from build123d import *

# Parameters (mm, degrees)
F0_W         = 177.8
F0_H         = 304.8
F1_DEPTH     = 762
F3_DEPTH     = 12.7
F5_T1_DEPTH  = 279.4
F5_T3_DEPTH  = 152.4
F5_T5_DEPTH  = 781.05
F5_T7_DEPTH  = 206.9983323097
F5_S11_W     = 12.954
F5_S11_H     = 12.954
F5_T12_DEPTH = 12.954
F5_S17_W     = 12.954
F5_S17_H     = 12.954
F5_T18_DEPTH = 12.954
F5_S23_W     = 12.954
F5_S23_H     = 12.954
F5_T24_DEPTH = 12.954
F5_S29_W     = 12.954
F5_S29_H     = 12.954
F5_T30_DEPTH = 12.954
F5_T34_ANGLE = 180
F5_T36_ANGLE = 180
F5_T38_ANGLE = 160.6620429302
F5_T40_ANGLE = 121.9975948725
F5_T42_ANGLE = 121.9975948725


# Not quite as in the source:
# - a fillet or chamfer that OpenCascade refuses, or shapes differently, is made with other operations: its cross-section is extruded or revolved along the edge and cut away or added
# - a feature of the source that left no trace in its solid (it failed there, or was rolled back) is left out


with BuildPart() as f1:
    # F0 (on Top) → F1 (new body)
    with BuildSketch(Plane.XY):
        Rectangle(F0_W, F0_H)
    extrude(amount=F1_DEPTH)

    # F2 (on face) → F3 (join)
    with BuildSketch(Plane.XZ.offset(152.4)):
        with BuildLine():
            ThreePointArc((0, 190.5), (-61.5022268, 124.3675088832), (-63.5, 34.0788651625))
            ThreePointArc((-63.5, 34.0788651625), (-36.0333838653, 9.0580961901), (3.12e-07, 0))
            ThreePointArc((3.12e-07, 0), (36.0333841402, 9.0580963377), (63.5, 34.0788651625))
            ThreePointArc((63.5, 34.0788651625), (61.5022268, 124.3675088832), (0, 190.5))
        make_face()
        with BuildLine():
            ThreePointArc((63.5, 685.8), (0, 749.3), (-63.5, 685.8))
            Line((-63.5, 685.8), (-63.5, 478.8016676903))
            ThreePointArc((-63.5, 478.8016676903), (0, 415.3016676903), (63.5, 478.8016676903))
            Line((63.5, 478.8016676903), (63.5, 685.8))
        make_face()
    extrude(amount=F3_DEPTH)

    # F5: fillet of radius 12.7 on 15 edges, made by hand

    # F5_s2 → F5_t1 (cut)
    with BuildSketch(Plane.XZ.offset(-139.7)):
        with BuildLine():
            ThreePointArc((88.9, 749.3), (85.1802561211, 758.2802561211), (76.2, 762))
            Line((76.2, 762), (88.9, 762))
            Line((88.9, 762), (88.9, 749.3))
        make_face()
        with BuildLine():
            ThreePointArc((-76.2, 762), (-85.1802561211, 758.2802561211), (-88.9, 749.3))
            Line((-88.9, 749.3), (-88.9, 762))
            Line((-88.9, 762), (-76.2, 762))
        make_face()
    extrude(amount=F5_T1_DEPTH, mode=Mode.SUBTRACT)

    # F5_s4 → F5_t3 (cut)
    with BuildSketch(Plane.YZ.offset(-76.2)):
        with BuildLine():
            ThreePointArc((152.4, 749.3), (148.6802561211, 758.2802561211), (139.7, 762))
            Line((139.7, 762), (152.4, 762))
            Line((152.4, 762), (152.4, 749.3))
        make_face()
        with BuildLine():
            ThreePointArc((-152.4, 749.3), (-148.6802561211, 758.2802561211), (-139.7, 762))
            Line((-139.7, 762), (-152.4, 762))
            Line((-152.4, 762), (-152.4, 749.3))
        make_face()
    extrude(amount=F5_T3_DEPTH, mode=Mode.SUBTRACT)

    # F5_s6 → F5_t5 (cut)
    with BuildSketch(Plane.XY.offset(-31.75)):
        with BuildLine():
            ThreePointArc((-76.2, -152.4), (-85.1802561211, -148.6802561211), (-88.9, -139.7))
            Line((-88.9, -139.7), (-88.9, -152.4))
            Line((-88.9, -152.4), (-76.2, -152.4))
        make_face()
        with BuildLine():
            ThreePointArc((-76.2, 152.4), (-85.1802561211, 148.6802561211), (-88.9, 139.7))
            Line((-88.9, 139.7), (-88.9, 152.4))
            Line((-88.9, 152.4), (-76.2, 152.4))
        make_face()
        with BuildLine():
            ThreePointArc((88.9, -139.7), (85.1802561211, -148.6802561211), (76.2, -152.4))
            Line((76.2, -152.4), (88.9, -152.4))
            Line((88.9, -152.4), (88.9, -139.7))
        make_face()
        with BuildLine():
            ThreePointArc((88.9, 139.7), (85.1802561211, 148.6802561211), (76.2, 152.4))
            Line((76.2, 152.4), (88.9, 152.4))
            Line((88.9, 152.4), (88.9, 139.7))
        make_face()
    extrude(amount=F5_T5_DEPTH, mode=Mode.SUBTRACT)

    # F5_s8 → F5_t7 (cut)
    with BuildSketch(Plane.XY.offset(478.8016676903)):
        with BuildLine():
            ThreePointArc((63.5, -152.4), (59.7802561211, -161.3802561211), (50.8, -165.1))
            Line((50.8, -165.1), (63.5, -165.1))
            Line((63.5, -165.1), (63.5, -152.4))
        make_face()
        with BuildLine():
            ThreePointArc((-63.5, -152.4), (-59.7802561211, -161.3802561211), (-50.8, -165.1))
            Line((-50.8, -165.1), (-63.5, -165.1))
            Line((-63.5, -165.1), (-63.5, -152.4))
        make_face()
    extrude(amount=F5_T7_DEPTH, mode=Mode.SUBTRACT)


with BuildPart() as f5_tool10:
    # F5_s11 → F5_t12 (new body)
    with BuildSketch(Plane.YZ.offset(76.2)):
        with Locations((-146.177, 755.777)):
            Rectangle(F5_S11_W, F5_S11_H)
    extrude(amount=F5_T12_DEPTH)

    # F5_s13 → F5_t14 (revolve, cut)
    with BuildSketch(Plane(origin=(76.2, -139.7, 749.3), x_dir=(0, 0.7071067812, -0.7071067812), z_dir=(0, -0.7071067812, -0.7071067812))):
        with BuildLine():
            ThreePointArc((0, -12.7), (12.7, 0), (0, 12.7))
            Line((0, 12.7), (0, -12.7))
        make_face()
    revolve(axis=Axis((76.2, -139.7, 749.3), (1, 0, 0)), mode=Mode.SUBTRACT)


with BuildPart() as f1_1:
    add(f1.part)

    # F5_t9: cut F5_tool10
    add(f5_tool10.part, mode=Mode.SUBTRACT)


with BuildPart() as f5_tool16:
    # F5_s17 → F5_t18 (new body)
    with BuildSketch(Plane.YZ.offset(76.2)):
        with Locations((146.177, 755.777)):
            Rectangle(F5_S17_W, F5_S17_H)
    extrude(amount=F5_T18_DEPTH)

    # F5_s19 → F5_t20 (revolve, cut)
    with BuildSketch(Plane(origin=(76.2, 139.7, 749.3), x_dir=(0, -0.7071067812, -0.7071067812), z_dir=(0, -0.7071067812, 0.7071067812))):
        with BuildLine():
            ThreePointArc((0, -12.7), (12.7, 0), (0, 12.7))
            Line((0, 12.7), (0, -12.7))
        make_face()
    revolve(axis=Axis((76.2, 139.7, 749.3), (1, 0, 0)), mode=Mode.SUBTRACT)


with BuildPart() as f1_2:
    add(f1_1.part)

    # F5_t15: cut F5_tool16
    add(f5_tool16.part, mode=Mode.SUBTRACT)


with BuildPart() as f5_tool22:
    # F5_s23 → F5_t24 (new body)
    with BuildSketch(Plane.XZ.offset(-139.7)):
        with Locations((-82.677, 755.777)):
            Rectangle(F5_S23_W, F5_S23_H)
    extrude(amount=-F5_T24_DEPTH)

    # F5_s25 → F5_t26 (revolve, cut)
    with BuildSketch(Plane(origin=(-76.2, 139.7, 749.3), x_dir=(0.7071067812, 0, -0.7071067812), z_dir=(0.7071067812, 0, 0.7071067812))):
        with BuildLine():
            ThreePointArc((0, -12.7), (12.7, 0), (0, 12.7))
            Line((0, 12.7), (0, -12.7))
        make_face()
    revolve(axis=Axis((-76.2, 139.7, 749.3), (0, 1, 0)), mode=Mode.SUBTRACT)


with BuildPart() as f1_3:
    add(f1_2.part)

    # F5_t21: cut F5_tool22
    add(f5_tool22.part, mode=Mode.SUBTRACT)


with BuildPart() as f5_tool28:
    # F5_s29 → F5_t30 (new body)
    with BuildSketch(Plane.XZ.offset(139.7)):
        with Locations((-82.677, 755.777)):
            Rectangle(F5_S29_W, F5_S29_H)
    extrude(amount=F5_T30_DEPTH)

    # F5_s31 → F5_t32 (revolve, cut)
    with BuildSketch(Plane(origin=(-76.2, -139.7, 749.3), x_dir=(0.7071067812, 0, -0.7071067812), z_dir=(-0.7071067812, 0, -0.7071067812))):
        with BuildLine():
            ThreePointArc((0, -12.7), (12.7, 0), (0, 12.7))
            Line((0, 12.7), (0, -12.7))
        make_face()
    revolve(axis=Axis((-76.2, -139.7, 749.3), (0, -1, 0)), mode=Mode.SUBTRACT)


with BuildPart() as f1_4:
    add(f1_3.part)

    # F5_t27: cut F5_tool28
    add(f5_tool28.part, mode=Mode.SUBTRACT)

    # F5_s33 → F5_t34 (revolve, cut)
    with BuildSketch(Plane.XY.offset(478.8016676903)):
        with BuildLine():
            ThreePointArc((-63.5, -152.4), (-59.7802561211, -161.3802561211), (-50.8, -165.1))
            Line((-50.8, -165.1), (-63.5, -165.1))
            Line((-63.5, -165.1), (-63.5, -152.4))
        make_face()
    revolve(axis=Axis((0, -165.1, 478.8016676903), (0, -1, 0)), revolution_arc=F5_T34_ANGLE, mode=Mode.SUBTRACT)

    # F5_s35 → F5_t36 (revolve, cut)
    with BuildSketch(Plane.XY.offset(685.8)):
        with BuildLine():
            ThreePointArc((63.5, -152.4), (59.7802561211, -161.3802561211), (50.8, -165.1))
            Line((50.8, -165.1), (63.5, -165.1))
            Line((63.5, -165.1), (63.5, -152.4))
        make_face()
    revolve(axis=Axis((0, -165.1, 685.8), (0, -1, 0)), revolution_arc=F5_T36_ANGLE, mode=Mode.SUBTRACT)

    # F5_s37 → F5_t38 (revolve, cut)
    with BuildSketch(Plane(origin=(-12.6164174444, 0, 74.050466073), x_dir=(0, 1, 0), z_dir=(-0.1679556687, 0, 0.9857945493))):
        with BuildLine():
            ThreePointArc((-152.4, 63.401778044), (-161.3802561211, 59.6820341651), (-165.1, 50.701778044))
            Line((-165.1, 50.701778044), (-165.1, 63.401778044))
            Line((-165.1, 63.401778044), (-152.4, 63.401778044))
        make_face()
    revolve(axis=Axis((0, -165.1, 76.2), (0, -1, 0)), revolution_arc=F5_T38_ANGLE, mode=Mode.SUBTRACT)

    # F5_s39 → F5_t40 (revolve, cut)
    with BuildSketch(Plane(origin=(69.2556243915, 0, 14.6214058217), x_dir=(0, 1, 0), z_dir=(0.9784320741, 0, 0.2065688173))):
        with BuildLine():
            ThreePointArc((-152.4, 190.3421366621), (-161.3802561211, 186.6223927832), (-165.1, 177.6421366621))
            Line((-165.1, 177.6421366621), (-165.1, 190.3421366621))
            Line((-165.1, 190.3421366621), (-152.4, 190.3421366621))
        make_face()
    revolve(axis=Axis((56.1711141332, -165.1, 76.5973839763), (0, -1, 0)), revolution_arc=F5_T40_ANGLE, mode=Mode.SUBTRACT)

    # F5_s41 → F5_t42 (revolve, cut)
    with BuildSketch(Plane(origin=(11.2454514703, 0, 11.6780216132), x_dir=(0, 1, 0), z_dir=(-0.6936400605, 0, -0.7203217798))):
        with BuildLine():
            ThreePointArc((-152.4, 33.4077090386), (-161.3802561211, 29.6879651596), (-165.1, 20.7077090386))
            Line((-165.1, 20.7077090386), (-165.1, 33.4077090386))
            Line((-165.1, 33.4077090386), (-152.4, 33.4077090386))
        make_face()
    revolve(axis=Axis((-56.1711141332, -165.1, 76.5973839763), (0, -1, 0)), revolution_arc=F5_T42_ANGLE, mode=Mode.SUBTRACT)


solid = f1_4.part
For this review, take the finished solid that the model builds, in its own axes (mm). A direction names the side the tool comes from. Round coordinates to 2 decimals unless told otherwise and drop trailing zeros. Loops run counter-clockwise (first coordinate to the right, second up) from the corner with the lowest first, then second, coordinate; pieces in that order, holes last. Notation, with made-up numbers: (81.25, 16.25) - (122.25, 16.25) arc R26 cw to (122.25, 42.25) - close; hole circle Ø3 at (61.5, -40). An arc over 180 degrees is marked (long way). Put each result on its own line as item: value. Start each with the question number.
1. For faces 1 (the cylindrical face through (-85.08, 1.96, 758.38)), 2 (the cylindrical face through (-59.88, -161.28, 580.85)), list the 3-axis set-ups (+Z, -Z, +X, -X, +Y, -Y) from which the entire face can be reached by the end or side of a thin tool; tool diameter is ignored.
2. Mouldability with a two-part tool opening along Z and no side actions: class faces 3 (the flat face through (-1, 2, 0)), 4 (the flat face through (-1, -152.4, 286)), 5 (the flat face through (-1, 2, 762)), 6 (the cylindrical face through (59.88, -161.28, 580.85)) as +Z half, -Z half, draft (parallel to the pull), parting line (faces both ways), or undercut.
3. Insertion check: P1, Ø5, axis at x = -52, z = 349.5, coming from the -Y side. The pin has a flat end and moves straight along its axis. Give the tip position at first contact, or say it passes through.
4. Consider section A-A on z = 588. State the section outline as (x, y) points, plus the area to 3 significant figures.
5. For probe 1 along Y at (x, z) = (52, 255.5); probe 2 along X at (y, z) = (-148.5, 427.5); probe 3 along Z at (x, y) = (-70, -147.5), list the stretches that pass through material, from the lowest coordinate up. Write a range as [from, to].
Result sheet:
1. face 1: +Z, -X, +Y, -Y
1. face 2: +Z, -X, -Y
2. face 3: -Z half
2. face 4: undercut
2. face 5: +Z half
2. face 6: draft
3. P1: y = -152.4
4. outline: (-88.9, -139.7) arc R12.7 ccw to (-76.2, -152.4) - (-63.5, -152.4) arc R12.7 ccw to (-50.8, -165.1) - (50.8, -165.1) arc R12.7 ccw to (63.5, -152.4) - (76.2, -152.4) arc R12.7 ccw to (88.9, -139.7) - (88.9, 139.7) arc R12.7 ccw to (76.2, 152.4) - (-76.2, 152.4) arc R12.7 ccw to (-88.9, 139.7) - close
4. area: 55,600 mm^2
5. probe 1: [-152.4, 152.4]
5. probe 2: [-85.36, 85.36]
5. probe 3: [0, 759.32]
